```python
from build123d import *

# Parameters (mm, degrees)
SKETCH1_R            = 2.0828
BOSS_EXTRUDE1_DEPTH  = 3
SKETCH2_W            = 20.32
SKETCH2_H            = 12.7
CUT_EXTRUDE1_DEPTH   = 99.104736331
SKETCH3_W            = 25.964797213
SKETCH3_H            = 13.829594426
SKETCH3_R            = 3.048
BOSS_EXTRUDE2_DEPTH  = 6
FILLET1_R            = 6
FILLET1_OF_MIRROR1_R = 6


with BuildPart() as part:
    # Sketch1 → Boss-Extrude1 (new, symmetric)
    with BuildSketch(Plane.XY):
        with BuildLine():
            Line((-82.07375, -16.66875), (19.52625, -16.66875))
            ThreePointArc((19.52625, -16.66875), (24.016378061, -18.528621939), (25.87625, -23.01875))
            Line((25.87625, -23.01875), (25.87625, -35.71875))
            ThreePointArc((25.87625, -35.71875), (24.016378061, -40.208878061), (19.52625, -42.06875))
            Line((19.52625, -42.06875), (-82.07375, -42.06875))
            ThreePointArc((-82.07375, -42.06875), (-86.563878061, -40.208878061), (-88.42375, -35.71875))
            Line((-88.42375, -35.71875), (-88.42375, -23.01875))
            ThreePointArc((-88.42375, -23.01875), (-86.563878061, -18.528621939), (-82.07375, -16.66875))
        make_face()
        with Locations((-82.07375, -23.01875)):
            Circle(SKETCH1_R, mode=Mode.SUBTRACT)
        with Locations((19.52625, -23.01875)):
            Circle(SKETCH1_R, mode=Mode.SUBTRACT)
        with Locations((-82.07375, -35.71875)):
            Circle(SKETCH1_R, mode=Mode.SUBTRACT)
        with Locations((19.52625, -35.71875)):
            Circle(SKETCH1_R, mode=Mode.SUBTRACT)
    extrude(amount=BOSS_EXTRUDE1_DEPTH, both=True)

    # Sketch2 → Cut-Extrude1 (cut, through all)
    with BuildSketch(Plane.XY.offset(3)):
        with Locations((-31.27375, -23.01875)):
            Rectangle(SKETCH2_W, SKETCH2_H)
    extrude(amount=-CUT_EXTRUDE1_DEPTH, mode=Mode.SUBTRACT)

    # Sketch3 → Boss-Extrude2 (add)
    with BuildSketch(Plane.XY.offset(3)):
        with Locations((-44.256148607, -48.983547213)):
            Rectangle(SKETCH3_W, SKETCH3_H)
        with Locations((-50.32375, -48.983547213)):
            Circle(SKETCH3_R, mode=Mode.SUBTRACT)
    boss_extrude2 = extrude(amount=-BOSS_EXTRUDE2_DEPTH)

    # Fillet1
    fillet1_edges = [part.edges().sort_by_distance(p)[0] for p in [
        (-57.238547213, -42.06875, 0),
        (-57.238547213, -55.898344426, 0),
    ]]
    fillet(fillet1_edges, radius=FILLET1_R)

    # Mirror1: Boss-Extrude2 across plane
    add(boss_extrude2.mirror(Plane(origin=(-31.27375, -55.898344426, -3), x_dir=(0, 0, 1), z_dir=(1, 0, 0))))

    # Fillet1 of Mirror1
    fillet1_of_mirror1_edges = [part.edges().sort_by_distance(p)[0] for p in [
        (-5.308952787, -42.06875, 0),
        (-5.308952787, -55.898344426, 0),
    ]]
    fillet(fillet1_of_mirror1_edges, radius=FILLET1_OF_MIRROR1_R)


solid = part.part
```
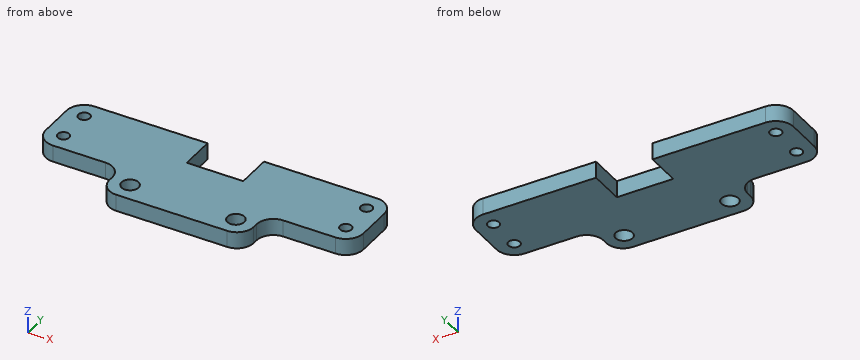
CAD build for the part. Positions are in the model's coordinates, mm. Round coordinates to 2 decimals unless told otherwise and drop trailing zeros. Write each loop counter-clockwise with the first axis right and the second up, starting at its lowest first coordinate (ties: lowest second). Pieces come first, ordered by that corner, then holes. Notation, with made-up numbers: (-6, 70.5) - (6, 70.5) arc R11 ccw to (6, 89.5) - close; hole circle Ø8 at (78, 83.5). An arc over 180 degrees is marked (long way). Return JSON: item names as keys, results as strings. Group by question number.
Item 1: Band-saw the part on A-A on z = -1.6. List the corners of the cut face in (x, y).
Item 2: Probe probe 1 along X at (y, z) = (-36, 0); probe 2 along Y at (x, z) = (-83, -1.75); probe 3 along Y at (x, z) = (18, -0.9). List the from-to ranges inside material, lowest first.
Item 3: Band-saw the part on B-B on x = -29. List the corners of the cut face in (y, z), plus the area to 3 significant figures.
Item 4: Band-saw the part on C-C on y = -44. List the corners of the cut face in (x, z), plus the area to 3 significant figures.
Item 5: Flat gauge pins, fed straight in: pin 1 Ø5 at (x, y) = (-82.07, -23.02) entering from +Z; pin 2 Ø1 at (y, z) = (-41, -2) entering from +X (3 decimals); pin 3 Ø3 at (x, z) = (-36, 0) entering from +Y; pin 4 Ø0.5 at (y, z) = (-49, -1) entering from +X. Where does each tip first touch, or does it go through?
Resolved:
{
 "1": {"outline": "(-88.42, -35.72) arc R6.35 ccw to (-82.07, -42.07) - (-63.24, -42.07) arc R6 cw to (-57.24, -48.07) - (-57.24, -49.9) arc R6 ccw to (-51.24, -55.9) - (-11.31, -55.9) arc R6 ccw to (-5.31, -49.9) - (-5.31, -48.07) arc R6 cw to (0.69, -42.07) - (19.53, -42.07) arc R6.35 ccw to (25.88, -35.72) - (25.88, -23.02) arc R6.35 ccw to (19.53, -16.67) - (-21.11, -16.67) - (-21.11, -29.37) - (-41.43, -29.37) - (-41.43, -16.67) - (-82.07, -16.67) arc R6.35 ccw to (-88.42, -23.02) - close; hole circle Ø4.17 at (-82.07, -35.72); hole circle Ø4.17 at (-82.07, -23.02); hole circle Ø6.1 at (-50.32, -48.98); hole circle Ø6.1 at (-12.22, -48.98); hole circle Ø4.17 at (19.53, -35.72); hole circle Ø4.17 at (19.53, -23.02)"},
 "2": {"probe 1": "x = -88.42 to -84.14, -80.01 to 17.46, 21.59 to 25.87", "probe 2": "y = -42 to -37.58, -33.85 to -24.88, -21.15 to -16.74", "probe 3": "y = -42.07 to -37.14, -34.3 to -24.44, -21.6 to -16.67"},
 "3": {"outline": "(-55.9, -3) - (-29.37, -3) - (-29.37, 3) - (-55.9, 3) - close", "area": "159 mm²"},
 "4": {"outline": "(-58.83, -3) - (-3.72, -3) - (-3.72, 3) - (-58.83, 3) - close", "area": "331 mm²"},
 "5": {"pin 1": "stops at z = 3", "pin 2": "stops at x = 23.705", "pin 3": "stops at y = -29.37", "pin 4": "stops at x = -5.31"}
}
